Geometry check sheet. Reference: the model listing, model coordinates, mm. A direction names the side the tool comes from. Coordinates: 2 decimals unless noted, no trailing zeros. Loops run counter-clockwise (first coordinate to the right, second up) from the corner with the lowest first, then second, coordinate; pieces in that order, holes last. Notation, with made-up numbers: M -10,67 L 25,67 A26 ccw 25,81 Z; hole C -32.5,-21 d2. An arc over 180 degrees is marked long. Use CSV: the item, a comma, the result in double quotes.
```python
from build123d import *

# Parameters (mm, degrees)
CROQUIS1_R              = 1.25
SALIENTE_EXTRUIR1_DEPTH = 2.5
CROQUIS2_R              = 55
CROQUIS2_R_2            = 40
SALIENTE_EXTRUIR3_DEPTH = 15
REDONDEO1_R             = 12
CROQUIS3_R              = 15
CROQUIS3_R_2            = 1.35
SALIENTE_EXTRUIR5_DEPTH = 5
CROQUIS4_R              = 4.3
CORTAR_EXTRUIR1_DEPTH   = 5


with BuildPart() as part:
    # Croquis1 → Saliente-Extruir1 (new body, symmetric)
    with BuildSketch(Plane.XY):
        with BuildLine():
            Line((-2, 44.955533586), (-2, 7.228416147))
            ThreePointArc((-2, 7.228416147), (-2.870125743, 6.929096494), (-3.697048513, 6.525475637))
            Line((-3.697048513, 6.525475637), (-30.374149088, 33.202576213))
            ThreePointArc((-30.374149088, 33.202576213), (-31.819805153, 31.819805153), (-33.202576213, 30.374149088))
            Line((-33.202576213, 30.374149088), (-6.525475637, 3.697048513))
            ThreePointArc((-6.525475637, 3.697048513), (-6.929096494, 2.870125743), (-7.228416147, 2))
            Line((-7.228416147, 2), (-44.955533586, 2))
            ThreePointArc((-44.955533586, 2), (-45, 0), (-44.955533586, -2))
            Line((-44.955533586, -2), (-7.228416147, -2))
            ThreePointArc((-7.228416147, -2), (-6.929096494, -2.870125743), (-6.525475637, -3.697048513))
            Line((-6.525475637, -3.697048513), (-33.202576213, -30.374149088))
            ThreePointArc((-33.202576213, -30.374149088), (-31.819805153, -31.819805153), (-30.374149088, -33.202576213))
            Line((-30.374149088, -33.202576213), (-3.697048513, -6.525475637))
            ThreePointArc((-3.697048513, -6.525475637), (-2.870125743, -6.929096494), (-2, -7.228416147))
            Line((-2, -7.228416147), (-2, -44.955533586))
            ThreePointArc((-2, -44.955533586), (0, -45), (2, -44.955533586))
            Line((2, -44.955533586), (2, -7.228416147))
            ThreePointArc((2, -7.228416147), (2.870125743, -6.929096494), (3.697048513, -6.525475637))
            Line((3.697048513, -6.525475637), (30.374149088, -33.202576213))
            ThreePointArc((30.374149088, -33.202576213), (31.819805153, -31.819805153), (33.202576213, -30.374149088))
            Line((33.202576213, -30.374149088), (6.525475637, -3.697048513))
            ThreePointArc((6.525475637, -3.697048513), (6.929096494, -2.870125743), (7.228416147, -2))
            Line((7.228416147, -2), (44.955533586, -2))
            ThreePointArc((44.955533586, -2), (44.988882023, -1.000247127), (45, 0))
            ThreePointArc((45, 0), (44.988882023, 1.000247127), (44.955533586, 2))
            Line((44.955533586, 2), (7.228416147, 2))
            ThreePointArc((7.228416147, 2), (6.929096494, 2.870125743), (6.525475637, 3.697048513))
            Line((6.525475637, 3.697048513), (33.202576213, 30.374149088))
            ThreePointArc((33.202576213, 30.374149088), (31.819805153, 31.819805153), (30.374149088, 33.202576213))
            Line((30.374149088, 33.202576213), (3.697048513, 6.525475637))
            ThreePointArc((3.697048513, 6.525475637), (2.870125743, 6.929096494), (2, 7.228416147))
            Line((2, 7.228416147), (2, 44.955533586))
            ThreePointArc((2, 44.955533586), (0, 45), (-2, 44.955533586))
        make_face()
        with Locations((0, -10)):
            Circle(CROQUIS1_R, mode=Mode.SUBTRACT)
        with Locations((-10, 0)):
            Circle(CROQUIS1_R, mode=Mode.SUBTRACT)
        with Locations((10, 0)):
            Circle(CROQUIS1_R, mode=Mode.SUBTRACT)
        with Locations((0, 10)):
            Circle(CROQUIS1_R, mode=Mode.SUBTRACT)
    extrude(amount=SALIENTE_EXTRUIR1_DEPTH, both=True)

    # Croquis2 → Saliente-Extruir3 (add, symmetric)
    with BuildSketch(Plane.XY):
        Circle(CROQUIS2_R)
        Circle(CROQUIS2_R_2, mode=Mode.SUBTRACT)
    extrude(amount=SALIENTE_EXTRUIR3_DEPTH, both=True)

    # Redondeo1
    redondeo1_edges = [part.edges().sort_by_distance(p)[0] for p in [
        (39.987490222, 1.000312842, -2.5),
        (28.284271247, 28.284271247, -2.5),
        (0, 40, -2.5),
        (-28.284271247, 28.284271247, -2.5),
        (-40, 0, -2.5),
        (-28.284271247, -28.284271247, -2.5),
        (0, -40, -2.5),
        (28.284271247, -28.284271247, -2.5),
        (28.284271247, -28.284271247, 2.5),
        (0, -40, 2.5),
        (-28.284271247, -28.284271247, 2.5),
        (-40, 0, 2.5),
        (-28.284271247, 28.284271247, 2.5),
        (0, 40, 2.5),
        (28.284271247, 28.284271247, 2.5),
        (39.987490222, 1.000312842, 2.5),
    ]]
    fillet(redondeo1_edges, radius=REDONDEO1_R)

    # Croquis3 → Saliente-Extruir5 (add)
    with BuildSketch(Plane(origin=(0, 0, -2.5), x_dir=(-1, 0, 0), z_dir=(0, 0, -1))):
        Circle(CROQUIS3_R)
        with Locations((0, 10)):
            Circle(CROQUIS3_R_2, mode=Mode.SUBTRACT)
        with Locations((10, 0)):
            Circle(CROQUIS3_R_2, mode=Mode.SUBTRACT)
        with Locations((0, -10)):
            Circle(CROQUIS3_R_2, mode=Mode.SUBTRACT)
        with Locations((-10, 0)):
            Circle(CROQUIS3_R_2, mode=Mode.SUBTRACT)
    extrude(amount=-SALIENTE_EXTRUIR5_DEPTH)

    # Croquis4 → Cortar-Extruir1 (cut)
    with BuildSketch(Plane.XY.offset(2.5)):
        Circle(CROQUIS4_R)
    extrude(amount=-CORTAR_EXTRUIR1_DEPTH, mode=Mode.SUBTRACT)


solid = part.part
```
1. Gauge pin test, flat ends, axial feed: P1, Ø10, axis at x = -25, z = -6, coming from the +Y side; P2, Ø4, axis at y = -12.5, z = 1, coming from the +X side; P3, Ø5, axis at y = 36.5, z = -5.5, coming from the -X side. Record the tip position at first contact, or that the pin passes through.
The answers:
P1,"y = 51.23"
P2,"x = 53.99"
P3,"x = -43.23"
2. Section check A-A, the plane x = 16.5. Record the cut outline in (y, z).
The answers:
outline,"M -52.47,-15 L -36.44,-15 L -36.44,15 L -52.47,15 Z; M -19.33,-2.5 L -13.67,-2.5 L -13.67,2.5 L -19.33,2.5 Z; M -2,-2.5 L 2,-2.5 L 2,2.5 L -2,2.5 Z; M 13.67,-2.5 L 19.33,-2.5 L 19.33,2.5 L 13.67,2.5 Z; M 36.44,-15 L 52.47,-15 L 52.47,15 L 36.44,15 Z"
3. Release check for a two-part mould opening along Y. For faces 1 (the cylindrical face through (-11.923, -53.692, 0.21)), 2 (the flat face through (4, -40, 15)), 3 (the cylindrical face through (-4.296, 0.189, 0.035)) record: +Y half, -Y half, draft (parallel to the pull), parting line (faces both ways), or undercut.
The answers:
face 1,"parting line"
face 2,"draft"
face 3,"undercut"
4. Set-up check for faces 4 (the flat face through (4, -40, -15)), 5 (the cylindrical face through (5.79, -13.837, -0.035)), 6 (the flat face through (0, 7, 2.5)): record each of +Z, -Z, +X, -X, +Y, -Y from which the full face is reachable in a straight line by a thin tool's end or side.
The answers:
face 4,"-Z, +X, -X, +Y, -Y"
face 5,"+Z, -Z"
face 6,"+Z"
5. Section check C-C, the plane x = 32. Count the separate pieces of the cut face and the enclosed holes in it, plus the area to 3 significant figures.
The answers:
separate pieces,"3"
enclosed holes,"0"
area,"1,270 mm^2"
6. Thickness scan on line 1 (Y direction, x = 0, z = -1.05); line 2 (Y direction, x = 26.5, z = -9); line 3 (Y direction, x = 8, z = 2). Record the ranges inside material, lowest first. Write a range as [from, to].
The answers:
line 1,"[-55, -11.25], [-8.75, -4.3], [4.3, 8.75], [11.25, 55]"
line 2,"[-48.19, -29.96], [-29.33, -28.16], [28.16, 29.33], [29.96, 48.19]"
line 3,"[-54.42, -39.19], [-12.69, 12.69], [39.19, 54.42]"
